from build123d import *

# Parameters (mm, degrees)
BOSS_EXTRUDE1_DEPTH = 20.32
CUT_EXTRUDE1_REACH  = 59.39


with BuildPart() as part:
    # Sketch1 → Boss-Extrude1 (new body)
    with BuildSketch(Plane.XY):
        with BuildLine():
            Line((0, 0), (30.734, 0))
            Line((30.734, 0), (30.734, 8.89))
            Line((30.734, 8.89), (31.840804573, 25.577359666))
            ThreePointArc((31.840804573, 25.577359666), (15.367, 43.18), (-1.106804573, 25.577359666))
            Line((-1.106804573, 25.577359666), (0, 8.89))
            Line((0, 8.89), (0, 0))
        make_face()
        with BuildLine():
            Line((3.181975953, 8.89), (27.552024047, 8.89))
            Line((27.552024047, 8.89), (28.02853988, 16.074458114))
            ThreePointArc((28.02853988, 16.074458114), (26.648414098, 14.615548708), (25.10136567, 13.335))
            Line((25.10136567, 13.335), (23.229372272, 15.899423077))
            ThreePointArc((23.229372272, 15.899423077), (15.367, 40.005), (7.504627728, 15.899423077))
            Line((7.504627728, 15.899423077), (5.63263433, 13.335))
            ThreePointArc((5.63263433, 13.335), (4.085585902, 14.615548708), (2.70546012, 16.074458114))
            Line((2.70546012, 16.074458114), (3.181975953, 8.89))
        make_face(mode=Mode.SUBTRACT)
    extrude(amount=BOSS_EXTRUDE1_DEPTH)

    # Sketch2 → Cut-Extrude1 (cut, up to next)
    with BuildSketch(Plane.XZ, mode=Mode.PRIVATE) as cut_extrude1_sk1:
        with BuildLine():
            Line((12.827, 12.2174), (17.907, 12.2174))
            ThreePointArc((17.907, 12.2174), (19.9644, 10.16), (17.907, 8.1026))
            Line((17.907, 8.1026), (12.827, 8.1026))
            ThreePointArc((12.827, 8.1026), (10.7696, 10.16), (12.827, 12.2174))
        make_face()
    cut_extrude1_tool1 = extrude(cut_extrude1_sk1.sketch, amount=-CUT_EXTRUDE1_REACH, mode=Mode.PRIVATE) & part.part
    add(cut_extrude1_tool1.solids().sort_by_distance((15.367, 0, 10.16))[0], mode=Mode.SUBTRACT)


solid = part.part
The listing builds one solid part. Answer for the finished solid, in the listing's coordinates (mm). A direction names the side the tool comes from. Coordinates: 2 decimals unless noted, no trailing zeros. Write each loop counter-clockwise with the first axis right and the second up, starting at its lowest first coordinate (ties: lowest second). Pieces come first, ordered by that corner, then holes. Notation, with made-up numbers: M -28.75,22 L 27.25,22 A20 ccw 27.25,30 Z; hole C 33.5,22.5 d8. An arc over 180 degrees is marked long. Use one line per item in the form item = value.
Item 1: Find section B-B, the plane x = 15. Give the vertices of the cut face in (y, z), plus the area to 3 significant figures.
Model answer:
outline = M 0,0 L 8.89,0 L 8.89,8.1 L 0,8.1 Z; M 0,12.22 L 8.89,12.22 L 8.89,20.32 L 0,20.32 Z; M 40,0 L 43.18,0 L 43.18,20.32 L 40,20.32 Z
area = 209 mm2
Item 2: The mould has two halves that part along X. Classify faces 4 (the face through (-0.56, 17.35, 10.02)), 5 (the face through (15, 4, 8.103)), 6 (the face through (31.28, 17.12, 10.02)): released by +X, released by -X, zero draft, split by the parting line, or undercut.
Model answer:
face_4 = released by -X
face_5 = undercut
face_6 = released by +X
Item 3: Given P1, Ø2, axis at y = 17.5, z = 13.5, coming from the +X side; P2, Ø7, axis at y = 4.5, z = 15, coming from the +X side; P3, Ø1.5, axis at y = 12, z = 12, coming from the -X side; P4, Ø4, axis at x = 16.5, y = 12, coming from the -Z side, each flat-ended and moving along its own axis, determine where each tip first touches the part or whether it passes through.
Model answer:
P1 = 31.37
P2 = 30.73
P3 = -0.26
P4 = through
Item 4: Find section D-D, the plane x = 20.5. Give the vertices of the cut face in (y, z), plus the area to 3 significant figures.
Model answer:
outline = M 0,0 L 8.89,0 L 8.89,20.32 L 0,20.32 Z; M 38.98,0 L 42.36,0 L 42.36,20.32 L 38.98,20.32 Z
area = 249 mm2
Item 5: Find the intervals of material crossed by probe 1 along X at (y, z) = (26.67, 16); probe 2 along Y at (x, z) = (6.5, 9.5); probe 3 along Y at (x, z) = (25, 17.5), in increasing order.
Model answer:
probe_1 = -1.14 to 2.03, 28.7 to 31.88
probe_2 = 0 to 8.89, 14.52 to 16.71, 36.63 to 40.6
probe_3 = 0 to 8.89, 13.47 to 17.45, 35.89 to 40.08
Item 6: For faces 1 (the face through (24.18, 14.6, 10.02)), 2 (the face through (19.964, 4.383, 10.205)), 3 (the face through (30.734, 4, 10)), determine the directions among +Z, -Z, +X, -X, +Y, -Y from which every point of the face is accessible in a straight line to the end or side of a thin tool.
Model answer:
face_1 = +Z, -Z
face_2 = -Y
face_3 = +Z, -Z, +X, -Y
Item 7: Find section C-C, the plane z = 10.16. Give the vertices of the cut face in (x, y) (3 decimals).
Model answer:
outline = M -1.107,25.577 L 0,8.89 L 0,0 L 10.77,0 L 10.77,8.89 L 3.182,8.89 L 2.705,16.074 A16.51 ccw 5.633,13.335 L 7.505,15.899 A13.335 cw long 23.229,15.899 L 25.101,13.335 A16.51 ccw 28.029,16.074 L 27.552,8.89 L 19.964,8.89 L 19.964,0 L 30.734,0 L 30.734,8.89 L 31.841,25.577 A16.51 ccw long Z
Item 8: Find section A-A, the plane y = 26.67. Give the vertices of the cut face in (x, z).
Model answer:
outline = M -1.14,0 L 2.03,0 L 2.03,20.32 L -1.14,20.32 Z; M 28.7,0 L 31.88,0 L 31.88,20.32 L 28.7,20.32 Z
